from build123d import *

# Parameters (mm, degrees)
F0_W     = 100
F0_H     = 30
F1_DEPTH = 30
F2_R     = 2.5
F3_DEPTH = 30
F4_R     = 5
F5_DEPTH = 100


with BuildPart() as f1:
    # F0 (on Top) → F1 (new body)
    with BuildSketch(Plane.XY):
        with Locations((50, 15)):
            Rectangle(F0_W, F0_H)
    extrude(amount=F1_DEPTH)

    # F2 (on face) → F3 (cut)
    with BuildSketch(Plane.XY.offset(30)):
        with Locations((50, 25)):
            Circle(F2_R)
    extrude(amount=-F3_DEPTH, mode=Mode.SUBTRACT)

    # F4 (on face) → F5 (cut)
    with BuildSketch(Plane.YZ.offset(100)):
        with Locations((15, 15)):
            Circle(F4_R)
    extrude(amount=-F5_DEPTH, mode=Mode.SUBTRACT)


solid = f1.part
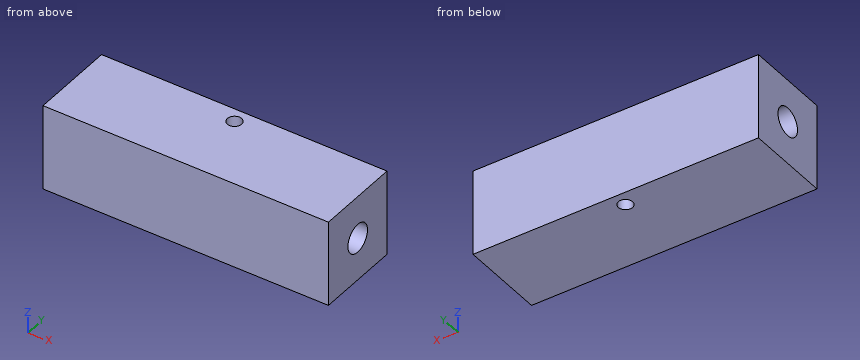
Part model, mm, in its own coordinate system. Round coordinates to 2 decimals unless told otherwise and drop trailing zeros. Write each loop counter-clockwise with the first axis right and the second up, starting at its lowest first coordinate (ties: lowest second). Pieces come first, ordered by that corner, then holes. Notation, with made-up numbers: M 53.5,85 L 58.5,85 A21 ccw 58.5,104 Z; hole C 44,-34 d11. An arc over 180 degrees is marked long. Return JSON: item names as keys, results as strings. Group by question number.
(1) Drill centre lines: probe 1 along X at (y, z) = (24.75, 21); probe 2 along Y at (x, z) = (50, 20.25); probe 3 along Y at (x, z) = (80.5, 15.25). Where is each one in solid material? Low to high.
(2) Saw through at C-C on x = 46. Write the cut outline in (y, z).
(3) Saw through at D-D on y = 15. Write the cut outline in (x, z), then the cut area to 3 significant figures.
(4) Saw through at B-B on y = 25. Write the cut outline in (x, z).
(5) Saw through at A-A on z = 15. Write the cut outline in (x, y), then the cut area to 3 significant figures.
Returned:
{
 "1": {"probe 1": "0 to 47.51, 52.49 to 100", "probe 2": "0 to 22.5, 27.5 to 30", "probe 3": "0 to 10.01, 19.99 to 30"},
 "2": {"outline": "M 0,0 L 30,0 L 30,30 L 0,30 Z; hole C 15,15 d10"},
 "3": {"outline": "M 0,0 L 100,0 L 100,10 L 0,10 Z; M 0,20 L 100,20 L 100,30 L 0,30 Z", "area": "2,000 mm²"},
 "4": {"outline": "M 0,0 L 47.5,0 L 47.5,30 L 0,30 Z; M 52.5,0 L 100,0 L 100,30 L 52.5,30 Z"},
 "5": {"outline": "M 0,0 L 100,0 L 100,10 L 0,10 Z; M 0,20 L 100,20 L 100,30 L 0,30 Z; hole C 50,25 d5", "area": "1,980 mm²"}
}
